Verification items for the finished model (mm, model axes). A direction names the side the tool comes from. Give positions to 0.01 mm unless a question says otherwise; leave off trailing zeros. Order: outer loops, then holes, each group sorted by start corner. A loop starts at its lowest first (then second) coordinate and runs counter-clockwise, first axis right, second up. Notation, with made-up numbers: (20, 24) -> (34, 24) arc R35 cw to (34, 61) -> close; hole circle Ø8 at (6.25, 7.5). An arc over 180 degrees is marked (long way). Return JSON: item names as keys, results as strings. Group by question number.
(1) Depth check by flat-ended pin: pin 1 Ø5 at (x, z) = (-0.5, -3) entering from +Y; pin 2 Ø1 at (y, z) = (-20, -1) entering from -X; pin 3 Ø1.5 at (y, z) = (-14, -2) entering from +X; pin 4 Ø2 at (x, z) = (0, 0) entering from +Y. Enter the tip coordinate at first touch or a pass-through.
(2) Thickness scan on line 1 along X through (y, z) = (1.05, 0); line 2 along Y through (x, z) = (3.25, 2.75); line 3 along Y through (x, z) = (-1.75, 0). Record the ranges inside material, lowest first.
(3) Release check for a two-part mould opening along Z. For faces 4 (the face through (-2.982, 1.972, 3.786)), 5 (the face through (4.475, 1.972, -1.788)), 6 (the face through (-3.786, 1.972, -2.982)), 7 (the face through (1, 4, -3)) record: pulls with the +Z half, pulls with the -Z half, needs draft (parallel to the pull), parting line crosses it, or undercut.
(4) Tool access check on faces 1 (the face through (0.7, 1.97, 4.79)), 2 (the face through (-4, 0, -1)), 3 (the face through (-1.788, 1.972, -4.475)). Record the directions out of +Z, -Z, +X, -X, +Y, -Y that give a thin tool (end or side, any length) a straight path to the whole face; none if there is none.
(5) Cross-section at A-A on y = -19. Enter the section's corners in (x, z), then the cut area to 3 significant figures.
from build123d import *

# Parameters (mm, degrees)
SKETCH1_R            = 5.5
SKETCH1_R_2          = 2
BOSS_EXTRUDE1_DEPTH  = 4
CUT_EXTRUDE1_DEPTH   = 4
FILLET1_R            = 0.2
FILLET2_R            = 0.4
FILLET1_OF_MIRROR1_R = 0.2
FILLET2_OF_MIRROR1_R = 0.4
CIRPATTERN1_DEPTH    = 4
SKETCH3_R            = 3
SKETCH3_R_2          = 2
BOSS_EXTRUDE2_DEPTH  = 0.5
CHAMFER1_SIZE        = 0.5
SKETCH4_R            = 3.5
BOSS_EXTRUDE3_DEPTH  = 1
SKETCH5_R            = 2.5
BOSS_EXTRUDE4_DEPTH  = 23


# Read off the part's stored shape, not the designer's step: CirPattern1
with BuildPart() as part:
    # Sketch1 → Boss-Extrude1 (new body)
    with BuildSketch(Plane(origin=(0, 0, 0), x_dir=(1, 0, 0), z_dir=(0, 1, 0))):
        with Locations(Location((0, 0, 0), (0, 0, 270))):
            Circle(SKETCH1_R)
        with Locations(Location((0, 0, 0), (0, 0, 270))):
            Circle(SKETCH1_R_2, mode=Mode.SUBTRACT)
    extrude(amount=BOSS_EXTRUDE1_DEPTH)

    # Sketch2 → Cut-Extrude1 (cut)
    with BuildSketch(Plane(origin=(0, 4, 0), x_dir=(1, 0, 0), z_dir=(0, 1, 0))):
        with BuildLine():
            Line((0, 3.799), (0, 7.477315916))
            Line((0, 7.477315916), (-1.717756705, 5.644784223))
            ThreePointArc((-1.717756705, 5.644784223), (-0.778860554, 4.915006115), (-0.449816676, 3.772275965))
            ThreePointArc((-0.449816676, 3.772275965), (-0.225304913, 3.792313106), (0, 3.799))
        make_face()
    cut_extrude1 = extrude(amount=-CUT_EXTRUDE1_DEPTH, mode=Mode.SUBTRACT)

    # Fillet1
    fillet1_edges = [part.edges().sort_by_distance(p)[0] for p in [
        (-1.205722077, 2, -5.366212284),
    ]]
    fillet(fillet1_edges, radius=FILLET1_R)

    # Fillet2
    fillet2_edges = [part.edges().sort_by_distance(p)[0] for p in [
        (-0.449816676, 2, -3.772275965),
    ]]
    fillet(fillet2_edges, radius=FILLET2_R)

    # Mirror1: Cut-Extrude1 across plane
    add(cut_extrude1.mirror(Plane.ZY), mode=Mode.SUBTRACT)

    # Fillet1 of Mirror1
    fillet1_of_mirror1_edges = [part.edges().sort_by_distance(p)[0] for p in [
        (1.205722077, 2, -5.366212284),
    ]]
    fillet(fillet1_of_mirror1_edges, radius=FILLET1_OF_MIRROR1_R)

    # Fillet2 of Mirror1
    fillet2_of_mirror1_edges = [part.edges().sort_by_distance(p)[0] for p in [
        (0.449816676, 2, -3.772275965),
    ]]
    fillet(fillet2_of_mirror1_edges, radius=FILLET2_OF_MIRROR1_R)

    # CirPattern1 outline → CirPattern1 (cut)
    with BuildSketch(Plane(origin=(0, 0, 0), x_dir=(1, 0, 0), z_dir=(0, 1, 0))):
        with BuildLine():
            ThreePointArc((3.62556251, 4.028637884), (3.71888228, 4.023485264), (3.799671329, 3.976493152))
            ThreePointArc((3.799671329, 3.976493152), (2.75, 4.76313972), (1.543908423, 5.278858473))
            ThreePointArc((1.543908423, 5.278858473), (1.62499931, 5.23238916), (1.676121495, 5.154148179))
            ThreePointArc((1.676121495, 5.154148179), (1.787762124, 4.48460755), (1.659448371, 3.81806133))
            ThreePointArc((1.659448371, 3.81806133), (1.656771541, 3.537498856), (1.839050027, 3.32419855))
            ThreePointArc((1.839050027, 3.32419855), (1.8995, 3.290030509), (1.959315378, 3.254763317))
            ThreePointArc((1.959315378, 3.254763317), (2.235178105, 3.203555671), (2.47681392, 3.34615511))
            ThreePointArc((2.47681392, 3.34615511), (2.989903003, 3.79055119), (3.62556251, 4.028637884))
        make_face()
        with BuildLine():
            ThreePointArc((5.154148179, 1.676121495), (5.23238916, 1.62499931), (5.278858473, 1.543908423))
            ThreePointArc((5.278858473, 1.543908423), (4.763139721, 2.75), (3.976493152, 3.799671329))
            ThreePointArc((3.976493152, 3.799671329), (4.023485264, 3.71888228), (4.028637884, 3.62556251))
            ThreePointArc((4.028637884, 3.62556251), (3.79055119, 2.989903003), (3.34615511, 2.47681392))
            ThreePointArc((3.34615511, 2.47681392), (3.203555671, 2.235178105), (3.254763317, 1.959315378))
            ThreePointArc((3.254763317, 1.959315378), (3.290030509, 1.8995), (3.32419855, 1.839050027))
            ThreePointArc((3.32419855, 1.839050027), (3.537498856, 1.656771541), (3.81806133, 1.659448371))
            ThreePointArc((3.81806133, 1.659448371), (4.48460755, 1.787762124), (5.154148179, 1.676121495))
        make_face()
        with BuildLine():
            ThreePointArc((5.301684005, -1.125510295), (5.34388159, -1.208903897), (5.343579752, -1.302365321))
            ThreePointArc((5.343579752, -1.302365321), (5.5, 0), (5.343579752, 1.302365321))
            ThreePointArc((5.343579752, 1.302365321), (5.34388159, 1.208903897), (5.301684005, 1.125510295))
            ThreePointArc((5.301684005, 1.125510295), (4.777665126, 0.69405636), (4.13626229, 0.47190622))
            ThreePointArc((4.13626229, 0.47190622), (3.891949646, 0.333943185), (3.798365405, 0.069435233))
            ThreePointArc((3.798365405, 0.069435233), (3.799, 0), (3.798365405, -0.069435233))
            ThreePointArc((3.798365405, -0.069435233), (3.891949646, -0.333943185), (4.13626229, -0.47190622))
            ThreePointArc((4.13626229, -0.47190622), (4.777665126, -0.69405636), (5.301684005, -1.125510295))
        make_face()
        with BuildLine():
            ThreePointArc((4.028637884, -3.62556251), (4.023485264, -3.71888228), (3.976493152, -3.799671329))
            ThreePointArc((3.976493152, -3.799671329), (4.763139721, -2.75), (5.278858473, -1.543908423))
            ThreePointArc((5.278858473, -1.543908423), (5.23238916, -1.62499931), (5.154148179, -1.676121495))
            ThreePointArc((5.154148179, -1.676121495), (4.48460755, -1.787762124), (3.81806133, -1.659448371))
            ThreePointArc((3.81806133, -1.659448371), (3.537498856, -1.656771541), (3.32419855, -1.839050027))
            ThreePointArc((3.32419855, -1.839050027), (3.290030509, -1.8995), (3.254763317, -1.959315378))
            ThreePointArc((3.254763317, -1.959315378), (3.203555671, -2.235178105), (3.34615511, -2.47681392))
            ThreePointArc((3.34615511, -2.47681392), (3.79055119, -2.989903003), (4.028637884, -3.62556251))
        make_face()
        with BuildLine():
            ThreePointArc((1.676121495, -5.154148179), (1.62499931, -5.23238916), (1.543908423, -5.278858473))
            ThreePointArc((1.543908423, -5.278858473), (2.75, -4.763139721), (3.799671329, -3.976493152))
            ThreePointArc((3.799671329, -3.976493152), (3.71888228, -4.023485264), (3.62556251, -4.028637884))
            ThreePointArc((3.62556251, -4.028637884), (2.989903003, -3.79055119), (2.47681392, -3.34615511))
            ThreePointArc((2.47681392, -3.34615511), (2.235178105, -3.203555671), (1.959315378, -3.254763317))
            ThreePointArc((1.959315378, -3.254763317), (1.8995, -3.290030509), (1.839050027, -3.32419855))
            ThreePointArc((1.839050027, -3.32419855), (1.656771541, -3.537498856), (1.659448371, -3.81806133))
            ThreePointArc((1.659448371, -3.81806133), (1.787762124, -4.48460755), (1.676121495, -5.154148179))
        make_face()
        with BuildLine():
            ThreePointArc((-1.125510295, -5.301684005), (-1.208903897, -5.34388159), (-1.302365321, -5.343579752))
            ThreePointArc((-1.302365321, -5.343579752), (0, -5.5), (1.302365321, -5.343579752))
            ThreePointArc((1.302365321, -5.343579752), (1.208903897, -5.34388159), (1.125510295, -5.301684005))
            ThreePointArc((1.125510295, -5.301684005), (0.69405636, -4.777665126), (0.47190622, -4.13626229))
            ThreePointArc((0.47190622, -4.13626229), (0.333943185, -3.891949646), (0.069435233, -3.798365405))
            ThreePointArc((0.069435233, -3.798365405), (0, -3.799), (-0.069435233, -3.798365405))
            ThreePointArc((-0.069435233, -3.798365405), (-0.333943185, -3.891949646), (-0.47190622, -4.13626229))
            ThreePointArc((-0.47190622, -4.13626229), (-0.69405636, -4.777665126), (-1.125510295, -5.301684005))
        make_face()
        with BuildLine():
            ThreePointArc((-3.62556251, -4.028637884), (-3.71888228, -4.023485264), (-3.799671329, -3.976493152))
            ThreePointArc((-3.799671329, -3.976493152), (-2.75, -4.763139721), (-1.543908423, -5.278858473))
            ThreePointArc((-1.543908423, -5.278858473), (-1.62499931, -5.23238916), (-1.676121495, -5.154148179))
            ThreePointArc((-1.676121495, -5.154148179), (-1.787762124, -4.48460755), (-1.659448371, -3.81806133))
            ThreePointArc((-1.659448371, -3.81806133), (-1.656771541, -3.537498856), (-1.839050027, -3.32419855))
            ThreePointArc((-1.839050027, -3.32419855), (-1.8995, -3.290030509), (-1.959315378, -3.254763317))
            ThreePointArc((-1.959315378, -3.254763317), (-2.235178105, -3.203555671), (-2.47681392, -3.34615511))
            ThreePointArc((-2.47681392, -3.34615511), (-2.989903003, -3.79055119), (-3.62556251, -4.028637884))
        make_face()
        with BuildLine():
            ThreePointArc((-5.154148179, -1.676121495), (-5.23238916, -1.62499931), (-5.278858473, -1.543908423))
            ThreePointArc((-5.278858473, -1.543908423), (-4.763139721, -2.75), (-3.976493152, -3.799671329))
            ThreePointArc((-3.976493152, -3.799671329), (-4.023485264, -3.71888228), (-4.028637884, -3.62556251))
            ThreePointArc((-4.028637884, -3.62556251), (-3.79055119, -2.989903003), (-3.34615511, -2.47681392))
            ThreePointArc((-3.34615511, -2.47681392), (-3.203555671, -2.235178105), (-3.254763317, -1.959315378))
            ThreePointArc((-3.254763317, -1.959315378), (-3.290030509, -1.8995), (-3.32419855, -1.839050027))
            ThreePointArc((-3.32419855, -1.839050027), (-3.537498856, -1.656771541), (-3.81806133, -1.659448371))
            ThreePointArc((-3.81806133, -1.659448371), (-4.48460755, -1.787762124), (-5.154148179, -1.676121495))
        make_face()
        with BuildLine():
            ThreePointArc((-5.301684005, 1.125510295), (-5.34388159, 1.208903897), (-5.343579752, 1.302365321))
            ThreePointArc((-5.343579752, 1.302365321), (-5.5, 0), (-5.343579752, -1.302365321))
            ThreePointArc((-5.343579752, -1.302365321), (-5.34388159, -1.208903897), (-5.301684005, -1.125510295))
            ThreePointArc((-5.301684005, -1.125510295), (-4.777665126, -0.69405636), (-4.13626229, -0.47190622))
            ThreePointArc((-4.13626229, -0.47190622), (-3.891949646, -0.333943185), (-3.798365405, -0.069435233))
            ThreePointArc((-3.798365405, -0.069435233), (-3.799, 0), (-3.798365405, 0.069435233))
            ThreePointArc((-3.798365405, 0.069435233), (-3.891949646, 0.333943185), (-4.13626229, 0.47190622))
            ThreePointArc((-4.13626229, 0.47190622), (-4.777665126, 0.69405636), (-5.301684005, 1.125510295))
        make_face()
        with BuildLine():
            ThreePointArc((-4.028637884, 3.62556251), (-4.023485264, 3.71888228), (-3.976493152, 3.799671329))
            ThreePointArc((-3.976493152, 3.799671329), (-4.763139721, 2.75), (-5.278858473, 1.543908423))
            ThreePointArc((-5.278858473, 1.543908423), (-5.23238916, 1.62499931), (-5.154148179, 1.676121495))
            ThreePointArc((-5.154148179, 1.676121495), (-4.48460755, 1.787762124), (-3.81806133, 1.659448371))
            ThreePointArc((-3.81806133, 1.659448371), (-3.537498856, 1.656771541), (-3.32419855, 1.839050027))
            ThreePointArc((-3.32419855, 1.839050027), (-3.290030509, 1.8995), (-3.254763317, 1.959315378))
            ThreePointArc((-3.254763317, 1.959315378), (-3.203555671, 2.235178105), (-3.34615511, 2.47681392))
            ThreePointArc((-3.34615511, 2.47681392), (-3.79055119, 2.989903003), (-4.028637884, 3.62556251))
        make_face()
        with BuildLine():
            ThreePointArc((-1.959315378, 3.254763317), (-1.8995, 3.290030509), (-1.839050027, 3.32419855))
            ThreePointArc((-1.839050027, 3.32419855), (-1.656771541, 3.537498856), (-1.659448371, 3.81806133))
            ThreePointArc((-1.659448371, 3.81806133), (-1.787762124, 4.48460755), (-1.676121495, 5.154148179))
            ThreePointArc((-1.676121495, 5.154148179), (-1.62499931, 5.23238916), (-1.543908423, 5.278858473))
            ThreePointArc((-1.543908423, 5.278858473), (-2.75, 4.76313972), (-3.799671329, 3.976493152))
            ThreePointArc((-3.799671329, 3.976493152), (-3.71888228, 4.023485264), (-3.62556251, 4.028637884))
            ThreePointArc((-3.62556251, 4.028637884), (-2.989903003, 3.79055119), (-2.47681392, 3.34615511))
            ThreePointArc((-2.47681392, 3.34615511), (-2.235178105, 3.203555671), (-1.959315378, 3.254763317))
        make_face()
    extrude(amount=CIRPATTERN1_DEPTH, mode=Mode.SUBTRACT)

    # Sketch3 → Boss-Extrude2 (add)
    with BuildSketch(Plane(origin=(0, 4, 0), x_dir=(1, 0, 0), z_dir=(0, 1, 0))):
        with Locations(Location((0, 0, 0), (0, 0, 270))):
            Circle(SKETCH3_R)
        with Locations(Location((0, 0, 0), (0, 0, 270))):
            Circle(SKETCH3_R_2, mode=Mode.SUBTRACT)
    extrude(amount=BOSS_EXTRUDE2_DEPTH)

    # Chamfer1
    chamfer1_edges = [part.edges().sort_by_distance(p)[0] for p in [
        (0, 4.5, -3),
    ]]
    chamfer(chamfer1_edges, length=CHAMFER1_SIZE - 0.0001)  # a hair under: the kernel refuses the full size

    # Sketch4 → Boss-Extrude3 (add)
    with BuildSketch(Plane.XZ):
        with Locations(Location((0, 0, 0), (0, 0, 90))):
            Circle(SKETCH4_R)
    extrude(amount=BOSS_EXTRUDE3_DEPTH)

    # Sketch5 → Boss-Extrude4 (add)
    with BuildSketch(Plane.XZ.offset(1)):
        with Locations(Location((0, 0, 0), (0, 0, 270))):
            Circle(SKETCH5_R)
    extrude(amount=BOSS_EXTRUDE4_DEPTH)


solid = part.part
Verdict:
{
 "1": {"pin 1": "y = 4.5", "pin 2": "x = -2.45", "pin 3": "x = 2.17", "pin 4": "y = 0"},
 "2": {"line 1": "-3.8 to -2, 2 to 3.8", "line 2": "0 to 4", "line 3": "-24 to 0"},
 "3": {"face 4": "pulls with the +Z half", "face 5": "undercut", "face 6": "undercut", "face 7": "needs draft"},
 "4": {"face 1": "+Z, +Y, -Y", "face 2": "-Y", "face 3": "+Y, -Y"},
 "5": {"outline": "circle Ø5 at (0, 0)", "area": "19.6 mm²"}
}
